The drawing under review shows one solid part. Ordinate dimensions are in mm from its lowest x, y, z. Round coordinates to 2 decimals unless told otherwise and drop trailing zeros. Write each loop counter-clockwise with the first axis right and the second up, starting at its lowest first coordinate (ties: lowest second). Pieces come first, ordered by that corner, then holes. Notation, with made-up numbers: (13, -4) -> (41, -4) arc R19 cw to (41, 23) -> close; hole circle Ø5 at (13, 52.5). An arc over 180 degrees is marked (long way). Use CSV: the item, a comma, the result in double quotes. Start each with the question number.
1) Take a section at C-C, the plane z = 3.6. Give the boundary of the cut face in (x, y), then the cut area to 3 significant figures.
2) For pin 1 Ø12 at (x, y) = (111, 19) entering from -Z; pin 2 Ø3 at (x, y) = (64.5, 17.5) entering from -Z, all flat-tipped, find the tip position at first contact; note any pin that passes through.
3) Take a section at A-A, the plane y = 25. Give the boundary of the cut face in (x, z).
4) Take a section at B-B, the plane x = 75. Give the boundary of the cut face in (y, z), then the cut area to 3 significant figures.
5) Wall thickness on probe 1 along X at (y, z) = (25, 2.1); probe 2 along Y at (x, z) = (75, 2.2); probe 3 along X at (y, z) = (27, 3.5): over which ranges is each line inside the solid? List them lowest first. Write a range as [from, to].
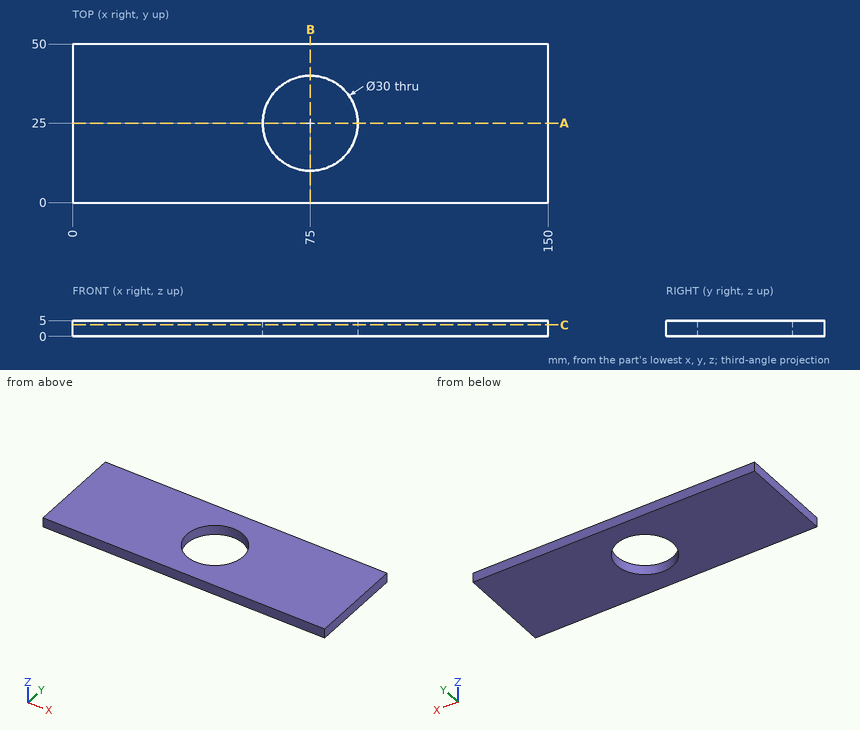
Values found:
1,outline,"(0, 0) -> (150, 0) -> (150, 50) -> (0, 50) -> close; hole circle Ø30 at (75, 25)"
1,area,"6,790 mm²"
2,pin 1,"z = 0"
2,pin 2,"through"
3,outline,"(0, 0) -> (60, 0) -> (60, 5) -> (0, 5) -> close; (90, 0) -> (150, 0) -> (150, 5) -> (90, 5) -> close"
4,outline,"(0, 0) -> (10, 0) -> (10, 5) -> (0, 5) -> close; (40, 0) -> (50, 0) -> (50, 5) -> (40, 5) -> close"
4,area,"100 mm²"
5,probe 1,"[0, 60], [90, 150]"
5,probe 2,"[0, 10], [40, 50]"
5,probe 3,"[0, 60.13], [89.87, 150]"
